from build123d import *

# Parameters (mm, degrees)
BASE_W                 = 22.25
BASE_H                 = 42.25
MAIN_DEPTH             = 3
GEAR_AXIS_HOLES_D      = 5.7
M1_6_CLEARANCE_HOLE1_D = 1.4
BOSS_EXTRUDE1_DEPTH    = 18.75
FILLET2_R              = 0.75
FILLET4_R              = 5
FILLET8_R              = 1.5
BOSS_EXTRUDE2_DEPTH    = 3
CHAMFER1_SIZE          = 3.5
FILLET6_R              = 3
CUT_EXTRUDE1_DEPTH     = 62.805259158
F_2_CLEARANCE_HOLE1_D  = 2.4384
M5_CLEARANCE_HOLE1_D   = 5.5
SKETCH20_W             = 18.125
SKETCH20_H             = 15
CUT_EXTRUDE2_DEPTH     = 18.75
FILLET7_R              = 5


with BuildPart() as part:
    # Base → Main (new body)
    with BuildSketch(Plane.XY):
        Polygon((-29.105845183, 40), (-29.105845183, -40), (-17.775845183, -40), (43.224154817, -40), (43.224154817, 40), align=None)
        with Locations((12.724154817, -8.375)):
            Rectangle(BASE_W, BASE_H, mode=Mode.SUBTRACT)
    extrude(amount=MAIN_DEPTH)

    # Gear Axis Holes (through all)
    with Locations(Plane(origin=(0, 0, 3), x_dir=(-1, 0, 0), z_dir=(0, 0, 1))):
        with Locations((22.605845183, 20), (22.605845183, -20)):
            Hole(GEAR_AXIS_HOLES_D / 2)

    # M1.6 Clearance Hole1 (through all)
    with Locations(Plane.XY.offset(3)):
        with Locations((17.724154817, -32.625), (7.724154817, -32.625), (7.724154817, 15.875), (17.724154817, 15.875)):
            Hole(M1_6_CLEARANCE_HOLE1_D / 2)

    # Sketch13 → Boss-Extrude1 (add)
    with BuildSketch(Plane.XY.offset(3)):
        Polygon((1.599154817, 30), (33.224154817, 30), (33.224154817, 1), (33.224154817, -30), (33.224154817, -40), (43.224154817, -40), (43.224154817, 1), (43.224154817, 40), (1.599154817, 40), align=None)
    extrude(amount=BOSS_EXTRUDE1_DEPTH)

    # Fillet2
    fillet2_edges = [part.edges().sort_by_distance(p)[0] for p in [
        (1.599154817, -29.5, 1.5),
        (23.849154817, -29.5, 1.5),
        (23.849154817, 12.75, 1.5),
        (1.599154817, 12.75, 1.5),
    ]]
    fillet(fillet2_edges, radius=FILLET2_R)

    # Fillet4
    fillet4_edges = [part.edges().sort_by_distance(p)[0] for p in [
        (1.599154817, 40, 12.375),
        (1.599154817, 30, 12.375),
        (33.224154817, 30, 12.375),
    ]]
    fillet(fillet4_edges, radius=FILLET4_R - 0.0001)  # a hair under: the kernel refuses the full size

    # Fillet8
    fillet8_edges = [part.edges().sort_by_distance(p)[0] for p in [
        (33.224154817, -40, 12.375),
    ]]
    fillet(fillet8_edges, radius=FILLET8_R)

    # Sketch21 → Boss-Extrude2 (add)
    with BuildSketch(Plane.XY.offset(3)):
        with BuildLine():
            Line((-29.105845183, 28.874119675), (-29.105845183, 11.125880325))
            ThreePointArc((-29.105845183, 11.125880325), (-33.605845183, 20), (-29.105845183, 28.874119675))
        make_face()
        with BuildLine():
            Line((-29.105845183, -11.125880325), (-29.105845183, -28.874119675))
            ThreePointArc((-29.105845183, -28.874119675), (-33.605845183, -20), (-29.105845183, -11.125880325))
        make_face()
    extrude(amount=-BOSS_EXTRUDE2_DEPTH)

    # Chamfer1
    chamfer1_edges = [part.edges().sort_by_distance(p)[0] for p in [
        (-29.105845183, -40, 1.5),
        (-29.105845183, 40, 1.5),
    ]]
    chamfer(chamfer1_edges, length=CHAMFER1_SIZE)

    # Fillet6
    fillet6_edges = [part.edges().sort_by_distance(p)[0] for p in [
        (-25.605845183, -40, 1.5),
        (-29.105845183, -36.5, 1.5),
        (-29.105845183, 36.5, 1.5),
        (-25.605845183, 40, 1.5),
        (43.224154817, 40, 10.875),
        (43.224154817, -40, 10.875),
    ]]
    fillet(fillet6_edges, radius=FILLET6_R)

    # Sketch14 → Cut-Extrude1 (cut, through all)
    with BuildSketch(Plane.XY.offset(3)):
        with BuildLine():
            Line((8.474154817, -33.325), (6.974154817, -33.325))
            ThreePointArc((6.974154817, -33.325), (6.274154817, -32.625), (6.974154817, -31.925))
            Line((6.974154817, -31.925), (8.474154817, -31.925))
            ThreePointArc((8.474154817, -31.925), (9.174154817, -32.625), (8.474154817, -33.325))
        make_face()
        with BuildLine():
            Line((18.474154817, -33.325), (16.974154817, -33.325))
            ThreePointArc((16.974154817, -33.325), (16.274154817, -32.625), (16.974154817, -31.925))
            Line((16.974154817, -31.925), (18.474154817, -31.925))
            ThreePointArc((18.474154817, -31.925), (19.174154817, -32.625), (18.474154817, -33.325))
        make_face()
        with BuildLine():
            Line((8.474154817, 16.575), (6.974154817, 16.575))
            ThreePointArc((6.974154817, 16.575), (6.274154817, 15.875), (6.974154817, 15.175))
            Line((6.974154817, 15.175), (8.474154817, 15.175))
            ThreePointArc((8.474154817, 15.175), (9.174154817, 15.875), (8.474154817, 16.575))
        make_face()
        with BuildLine():
            Line((18.474154817, 16.575), (16.974154817, 16.575))
            ThreePointArc((16.974154817, 16.575), (16.274154817, 15.875), (16.974154817, 15.175))
            Line((16.974154817, 15.175), (18.474154817, 15.175))
            ThreePointArc((18.474154817, 15.175), (19.174154817, 15.875), (18.474154817, 16.575))
        make_face()
    extrude(amount=-CUT_EXTRUDE1_DEPTH, mode=Mode.SUBTRACT)

    # #2 Clearance Hole1 (through all)
    with Locations(Plane.XY.offset(21.75)):
        with Locations((9.099154817, 35), (38.224154817, 35), (38.224154817, -35)):
            Hole(F_2_CLEARANCE_HOLE1_D / 2)

    # M5 Clearance Hole1 (through all)
    with Locations(Plane.ZY.offset(-33.224154817)):
        with Locations((9.25, 20), (9.25, -33.5)):
            Hole(M5_CLEARANCE_HOLE1_D / 2)

    # Sketch20 → Cut-Extrude2 (cut)
    with BuildSketch(Plane.XY.offset(21.75)):
        with Locations((24.161654817, 32.5)):
            Rectangle(SKETCH20_W, SKETCH20_H)
    extrude(amount=-CUT_EXTRUDE2_DEPTH, mode=Mode.SUBTRACT)

    # Fillet7
    fillet7_edges = [part.edges().sort_by_distance(p)[0] for p in [
        (15.099154817, 40, 12.375),
        (15.099154817, 30, 12.375),
    ]]
    fillet(fillet7_edges, radius=FILLET7_R - 0.0001)  # a hair under: the kernel refuses the full size


solid = part.part
The listing builds one solid part. Answer for the finished solid, in the listing's coordinates (mm). A direction names the side the tool comes from. Give positions to 0.01 mm unless a question says otherwise; leave off trailing zeros. Order: outer loops, then holes, each group sorted by start corner. A loop starts at its lowest first (then second) coordinate and runs counter-clockwise, first axis right, second up. Notation, with made-up numbers: (-20, -25.5) - (-14, -25.5) arc R21 ccw to (-14, 11.5) - close; hole circle Ø3 at (27, 69.25). An arc over 180 degrees is marked (long way). One line per item, written item: value. Start each with the question number.
1) Given pin 1 Ø4 at (x, y) = (-19, 6.5) entering from +Z; pin 2 Ø1.5 at (y, z) = (33.5, 2) entering from -X; pin 3 Ø10 at (y, z) = (29, 13) entering from -X, each flat-ended and moving along its own axis, determine where each tip first touches the part or whether it passes through.
2) The mould has two halves that part along Y. Classify faces 1 (the face through (38.294, -30.773, 9.608)), 2 (the face through (-25.526, 39.765, 1.521)), 3 (the face through (13.67, 31.5, 12.24)): released by +Y, released by -Y, zero draft, split by the parting line, or undercut.
3) A cutting plane is placed at D-D on y = 20. Give the vertices of the cut face in (x, z).
4) Find the intervals of material crossed by L1, parallel to X at y = -20, z = 0.7; L2, parallel to Y at x = 39.5, z = 9.25; L3, parallel to X at y = 9, z = 1.5, in increasing order.
5) A cutting plane is placed at A-A on y = 10. Give the vertices of the cut face in (x, z), then the cut area to 3 significant figures.
6) A cutting plane is placed at C-C on z = 1.5. State how many separate pieces and enclosed holes the cut face has, then the cut area to 3 significant figures.
7) A tool of negligible diameter and unlimited length cuts with its end or side. For faces 4 (the face through (13.6, 38.57, 12.24)), 5 (the face through (-29.106, 0, 1)), 6 (the face through (3.025, 31.504, 12.506)), 7 (the face through (1.599, -9, 1)), from which of +Z, -Z, +X, -X, +Y, -Y can it reach the whole face along a straight path? Write none if from no direction.
8) A cutting plane is placed at B-B on y = -20. Give the vertices of the cut face in (x, z).
Answer sheet:
1. pin 1: stops at z = 3
1. pin 2: stops at x = -29.11
1. pin 3: stops at x = 1.7
2. face 1: undercut
2. face 2: released by +Y
2. face 3: released by -Y
3. outline: (-33.61, 0) - (-25.46, 0) - (-25.46, 3) - (-33.61, 3) - close; (-19.76, 0) - (43.22, 0) - (43.22, 6.5) - (33.22, 6.5) - (33.22, 3) - (-19.76, 3) - close; (33.22, 12) - (43.22, 12) - (43.22, 21.75) - (33.22, 21.75) - close
4. L1: x = -33.61 to -25.46, -19.76 to 1.6, 23.85 to 43.22
4. L2: y = -40 to -36.25, -30.75 to 17.25, 22.75 to 40
4. L3: x = -29.11 to 1.6, 23.85 to 43.22
5. outline: (-29.11, 0) - (1.6, 0) - (1.6, 3) - (-29.11, 3) - close; (23.85, 0) - (43.22, 0) - (43.22, 21.75) - (33.22, 21.75) - (33.22, 3) - (23.85, 3) - close
5. area: 338 mm2
6. separate pieces: 1
6. enclosed holes: 10
6. area: 4,860 mm2
7. face 4: +Z, +Y
7. face 5: +Z, -Z, -X
7. face 6: +Z, -X, -Y
7. face 7: +Z, -Z
8. outline: (-33.61, 0) - (-25.46, 0) - (-25.46, 3) - (-33.61, 3) - close; (-19.76, 0) - (1.6, 0) - (1.6, 3) - (-19.76, 3) - close; (23.85, 0) - (43.22, 0) - (43.22, 21.75) - (33.22, 21.75) - (33.22, 3) - (23.85, 3) - close
